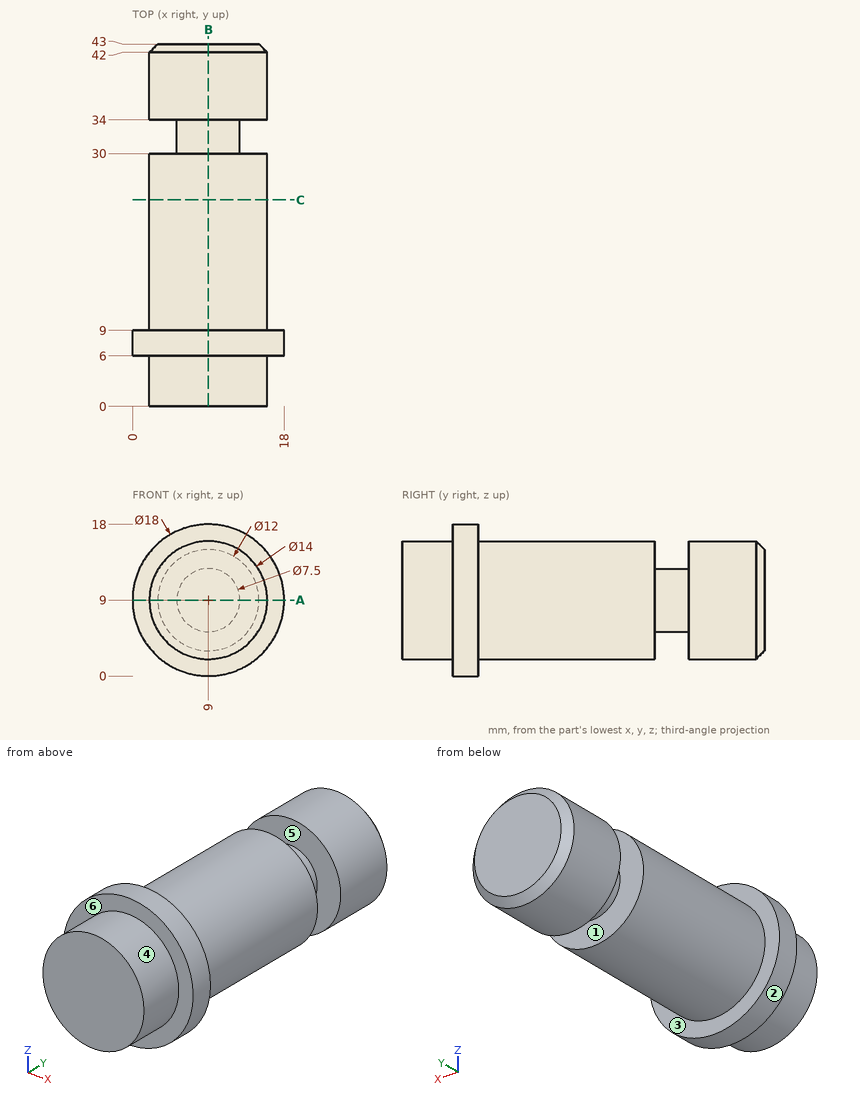
Here's the drawing with two shaded views (mm, measured from the low corner). I have some questions. A direction names the side the tool comes from. Round coordinates to 2 decimals unless told otherwise and drop trailing zeros. Order: outer loops, then holes, each group sorted by start corner. A loop starts at its lowest first (then second) coordinate and runs counter-clockwise, first axis right, second up. Notation, with made-up numbers: (-17.75, 60.25) -> (4.25, 60.25) arc R23 ccw to (4.25, 91.25) -> close; hole circle Ø7 at (-26.5, 23). An arc over 180 degrees is marked (long way). Write each question's results on one line, items separated by ' | '. Start each with the question number.
Item 1: Please list where these lines run through material, in increasing order: L1, parallel to Y at x = 7.5, z = 5.5; L2, parallel to Y at x = 2.5, z = 12; L3, parallel to Z at x = 8.75, y = 26.5.
Item 2: If we section it at A-A, the plane z = 9: Write out the boundary of the cut face in (x, y).
Item 3: Which directions (+Z, -Z, +X, -X, +Y, -Y) give clear straight access to the entire face, cutting with the end or side of a thin tool? Please do the marked faces 1, 2 and 3.
Item 4: If we section it at B-B, the plane x = 9: Write out the boundary of the cut face in (y, z), then the cut area to 3 significant figures.
Item 5: Thinking about a two-plate mould opening in Y: for the marked faces 4, 5 and 6, which applies, +Y half, -Y half, draft (parallel to the pull), parting line (faces both ways), or undercut?
Item 6: Will these pins go through, and if not, where does the flat tip stop? pin 1 (5 mm diameter, centred on y = 21, z = 11.5, fed in from -X); pin 2 (1 mm diameter, centred on x = 9.5, y = 12, fed in from +Z); pin 3 (2 mm diameter, centred on x = 3.5, y = 22, fed in from +Z).
Item 7: If we section it at C-C, the plane y = 24.5: Write out the boundary of the cut face in (x, z), then the cut area to 3 significant figures.
Results:
1) L1: y = 0 to 30, 34 to 43 | L2: y = 6 to 9 | L3: z = 2 to 16
2) outline: (0, 6) -> (2, 6) -> (2, 0) -> (16, 0) -> (16, 6) -> (18, 6) -> (18, 9) -> (16, 9) -> (16, 30) -> (12.75, 30) -> (12.75, 34) -> (16, 34) -> (16, 42) -> (15, 43) -> (3, 43) -> (2, 42) -> (2, 34) -> (5.25, 34) -> (5.25, 30) -> (2, 30) -> (2, 9) -> (0, 9) -> close
3) face 1: none | face 2: +Y, -Y | face 3: +Y
4) outline: (0, 2) -> (6, 2) -> (6, 0) -> (9, 0) -> (9, 2) -> (30, 2) -> (30, 5.25) -> (34, 5.25) -> (34, 2) -> (42, 2) -> (43, 3) -> (43, 15) -> (42, 16) -> (34, 16) -> (34, 12.75) -> (30, 12.75) -> (30, 16) -> (9, 16) -> (9, 18) -> (6, 18) -> (6, 16) -> (0, 16) -> close | area: 587 mm2
5) face 4: draft | face 5: undercut | face 6: -Y half
6) pin 1: stops at x = 2 | pin 2: stops at z = 16 | pin 3: stops at z = 14.36
7) outline: circle Ø14 at (9, 9) | area: 154 mm2
